Autodesk Inventor part; units mm, degrees
ref_plane "YZ Plane" through (0, 0, 0) normal (1, 0, 0) x (0, 1, 0)
ref_plane "XZ Plane" through (0, 0, 0) normal (0, 1, 0) x (-1, 0, 0)
ref_plane "XY Plane" through (0, 0, 0) normal (0, 0, 1) x (1, 0, 0)
sketch "Sketch1" plane through (0, 0, 0) normal (0, 0, 1) x (1, 0, 0)
  circle A0 centre (0, 0) radius 11.25
  circle A1 centre (0, 0) radius 37.0304
  arc A2 (-32.7929, -17.201) -> (-31.2929, -19.799) centre (0, 0) ccw
  line L0 (-32.7929, -17.201) -> (-31.0547, -16.1974)
  line L1 (-32.7929, -17.201) -> (-31.0547, -16.1974)
  line L2 (-29.5547, -18.7955) -> (-31.2929, -19.799)
  line L3 (-31.2929, -19.799) -> (-29.5547, -18.7955)
  line L4 (-16.1974, -31.0547) -> (-17.201, -32.7929)
  line L5 (-17.201, -32.7929) -> (-16.1974, -31.0547)
  arc A3 (-19.799, -31.2929) -> (-17.201, -32.7929) centre (0, 0) ccw
  line L6 (-19.799, -31.2929) -> (-18.7955, -29.5547)
  line L7 (-19.799, -31.2929) -> (-18.7955, -29.5547)
  arc A4 (17.201, -32.7929) -> (19.799, -31.2929) centre (0, 0) ccw
  line L8 (17.201, -32.7929) -> (16.1974, -31.0547)
  line L9 (17.201, -32.7929) -> (16.1974, -31.0547)
  line L10 (18.7955, -29.5547) -> (19.799, -31.2929)
  line L11 (19.799, -31.2929) -> (18.7955, -29.5547)
  arc A5 (31.2929, -19.799) -> (32.7929, -17.201) centre (0, 0) ccw
  line L12 (31.2929, -19.799) -> (29.5547, -18.7955)
  line L13 (31.0547, -16.1974) -> (32.7929, -17.201)
  line L14 (32.7929, -17.201) -> (31.0547, -16.1974)
  line L15 (32.7929, 17.201) -> (31.0547, 16.1974)
  line L16 (32.7929, 17.201) -> (31.0547, 16.1974)
  arc A6 (32.7929, 17.201) -> (31.2929, 19.799) centre (0, 0) ccw
  line L17 (29.5547, 18.7955) -> (31.2929, 19.799)
  line L18 (31.2929, 19.799) -> (29.5547, 18.7955)
  line L19 (16.1974, 31.0547) -> (17.201, 32.7929)
  line L20 (17.201, 32.7929) -> (16.1974, 31.0547)
  line L21 (19.799, 31.2929) -> (18.7955, 29.5547)
  line L22 (19.799, 31.2929) -> (18.7955, 29.5547)
  line L23 (-17.201, 32.7929) -> (-16.1974, 31.0547)
  line L24 (-17.201, 32.7929) -> (-16.1974, 31.0547)
  line L25 (-18.7955, 29.5547) -> (-19.799, 31.2929)
  line L26 (-19.799, 31.2929) -> (-18.7955, 29.5547)
  arc A7 (-31.2929, 19.799) -> (-32.7929, 17.201) centre (0, 0) ccw
  line L27 (-31.2929, 19.799) -> (-29.5547, 18.7955)
  line L28 (-31.2929, 19.799) -> (-29.5547, 18.7955)
  line L29 (-31.0547, 16.1974) -> (-32.7929, 17.201)
  line L30 (-32.7929, 17.201) -> (-31.0547, 16.1974)
  arc A8 (-21.806, -27.4089) -> (-27.4089, -21.806) centre (-22.4506, -22.4506) ccw
  circle A9 centre (-31.75, 0) radius 5
  arc A10 (-3.9618, 34.8002) -> (-2.3096, 31.8679) centre (-22.4506, 22.4506) ccw
  circle A11 centre (-22.4506, 22.4506) radius 5
  circle A12 centre (22.4506, 22.4506) radius 5
  circle A13 centre (22.4506, 22.4506) radius 5
  arc A14 (-3.9618, -34.8002) -> (-1.7951, -38.6456) centre (22.4506, -22.4506) ccw
  circle A15 centre (22.4506, -22.4506) radius 5
  circle A16 centre (-22.4506, 22.4506) radius 4.75
  circle A17 centre (-22.4506, -22.4506) radius 4.75
  circle A18 centre (22.4506, -22.4506) radius 4.75
  circle A19 centre (22.4506, 22.4506) radius 4.75
  circle A20 centre (0, 0) radius 34.775
  circle A21 centre (0, 0) radius 36.75
  point P0 (0, 0)
  point P1 (0, 49.75)
  point P2 (27.1463, 21.7343)
  point P3 (21.7343, 27.1463)
  point P4 (-21.7343, 27.1463)
  point P5 (-27.1463, 21.7343)
  point P6 (-27.1463, -21.7343)
  point P7 (-21.7343, -27.1463)
  point P8 (21.7343, -27.1463)
  point P9 (27.1463, -21.7343)
  dimension "d6" = 70.05
  dimension "d8" = 74.0608
  dimension "d0" = 10
  dimension "d1" = 0.25
  dimension "d4" = 360
  dimension "d7" = 0.25
  dimension "d9" = 73.5
extrude "Extrusion1" add sketch "Sketch1" along normal blind 21.9 contours A0 A10 | A9 A20 A11 A12 A15 A8 | A9 A20 A10 | A10 A20 A9 | A10 A0 | A20 A16 A11 | A8 A20 A17 | A20 A16 | A16 A20 | A20 A17 | A17 A20 | A15 A20 A18 | A20 A19 A12 | A20 A18 | A18 A20 | A20 A19 | A19 A20 picked at (-31.3962, -1.5997) picked at (-30.2693, 2.6951) picked at (-26.6756, 20.1619) picked at (20.1869, -26.6901) picked at (20.1869, 26.6901)
sketch "Skizze6" plane through (0, 0, 21.9) normal (0, 0, 1) x (1, 0, 0)
  circle A0 centre (0, 0) radius 12.225
  dimension "d33" = 24.45
extrude "Extrusion6" cut sketch "Skizze6" against normal through all
sketch "Skizze7" plane through (0, 0, 21.9) normal (0, 0, 1) x (1, 0, 0)
  line L0 (0, 0) -> (0, 1.75)
  line L1 (-25.23, 24.52) -> (25.23, 24.52)
  line L2 (25.23, 24.52) -> (25.23, -21.02)
  line L3 (25.23, -21.02) -> (-25.23, -21.02)
  line L4 (-25.23, -21.02) -> (-25.23, 24.52)
  line L5 (-25.23, 24.52) -> (25.23, -21.02) construction
  line L6 (25.23, 24.52) -> (-25.23, -21.02) construction
  dimension "d48" = 1.75
  dimension "d49" = 50.46
  dimension "d50" = 45.54
extrude "Extrusion7" cut sketch "Skizze7" against normal blind 7.4
sketch "Skizze8" plane through (0, 0, 0) normal (0, 0, -1) x (-1, 0, 0)
  circle A0 centre (0, 0) radius 12.225
  line L0 (-11.57, 11.47) -> (11.57, 11.47)
  line L1 (11.57, 11.57) -> (11.57, -11.57)
  line L2 (11.57, -11.57) -> (-11.57, -11.57)
  line L3 (-11.57, -11.57) -> (-11.57, 11.57)
  line L4 (-11.57, 11.57) -> (11.57, -11.57) construction
  line L5 (11.57, 11.57) -> (-11.57, -11.57) construction
  circle A1 centre (-11.57, 11.47) radius 1.75
  circle A2 centre (11.57, 11.47) radius 1.75
  circle A3 centre (11.57, -11.57) radius 1.75
  circle A4 centre (-11.57, -11.57) radius 1.75
  dimension "d40" = 23.14
  dimension "d41" = 23.14
  dimension "d42" = 3.5
  dimension "d43" = 3.5
  dimension "d44" = 3.5
  dimension "d45" = 3.5
extrude "Extrusion8" cut sketch "Skizze8" against normal through all contours A2 L0 L1 | L1 L0 A2 | A3 L2 L1 | L1 L2 A3 | A1 L3 L0 | L0 L3 A1 | A4 L3 L2 | L2 L3 A4
sketch "Skizze9" plane through (0, 0, 0) normal (0, 0, -1) x (-1, 0, 0)
  circle A0 centre (-11.57, 11.47) radius 1.75
  circle A1 centre (11.57, 11.47) radius 1.75
  circle A2 centre (11.57, -11.57) radius 1.75
  circle A3 centre (-11.57, -11.57) radius 1.75
  circle A4 centre (-11.57, 11.47) radius 3.1
  circle A5 centre (11.57, 11.47) radius 3.1
  circle A6 centre (11.57, -11.57) radius 3.1
  circle A7 centre (-11.57, -11.57) radius 3.1
  point P0 (0, 0)
  dimension "d51" = 6.2
  dimension "d52" = 6.2
  dimension "d53" = 6.2
  dimension "d54" = 6.2
extrude "Extrusion9" cut sketch "Skizze9" against normal blind 3.5 contours A0 | A1 | A2 | A3 | A4 | A5 | A6 | A7
properties part number "2024_08_26_beam_combiner_blende"
Verification items for the finished model (mm, model axes). A direction names the side the tool comes from. Coordinates: 2 decimals unless noted, no trailing zeros. Write each loop counter-clockwise with the first axis right and the second up, starting at its lowest first coordinate (ties: lowest second). Pieces come first, ordered by that corner, then holes. Notation, with made-up numbers: (80, -31.75) - (97, -31.75) arc R16 ccw to (97, -24.75) - close; hole circle Ø2 at (87, 20.5). An arc over 180 degrees is marked (long way). Write item = value, one per line.
Q1. Cross-section at C-C (x = 0). Enter the section's corners in (y, z) (3 decimals).
Answer:
outline = (-34.775, 0) - (-12.225, 0) - (-12.225, 14.5) - (-21.02, 14.5) - (-21.02, 21.9) - (-34.775, 21.9) - close; (12.225, 0) - (34.775, 0) - (34.775, 21.9) - (24.52, 21.9) - (24.52, 14.5) - (12.225, 14.5) - close
Q2. Cross-section at D-D (z = 16.75). Enter the section's corners in (x, y) (3 decimals), plus the area to 3 significant figures.
Answer:
outline = (-27.146, -21.734) arc R4.75 ccw to (-21.734, -27.146) arc R34.775 ccw to (21.734, -27.146) arc R4.75 ccw to (27.146, -21.734) arc R34.775 ccw to (27.146, 21.734) arc R4.75 ccw to (21.734, 27.146) arc R34.775 ccw to (-21.734, 27.146) arc R4.75 ccw to (-27.146, 21.734) arc R34.775 ccw to start; hole (-25.23, -21.02) - (25.23, -21.02) - (25.23, 24.52) - (-25.23, 24.52) - close
area = 1,540 mm²
Q3. Access from +Z, -Z, +X, -X, +Y, -Y to the whole of each face (thin tool, end or side, straight path). Record for faces 1 (the face through (0, -23, 21.9)), 2 (the face through (10.14, 8.72, 1.73)), 3 (the face through (0, -21.02, 18)).
Answer:
face_1 = +Z, +X, -X, +Y, -Y
face_2 = -Z
face_3 = +Z
Q4. Cross-section at A-A (y = 0). Enter the section's corners in (x, z) (3 decimals), plus the area to 3 significant figures.
Answer:
outline = (-34.775, 0) - (-12.225, 0) - (-12.225, 14.5) - (-25.23, 14.5) - (-25.23, 21.9) - (-34.775, 21.9) - close; (12.225, 0) - (34.775, 0) - (34.775, 21.9) - (25.23, 21.9) - (25.23, 14.5) - (12.225, 14.5) - close
area = 795 mm²
Q5. Go/stop test with flat-tipped pins: pin 1 Ø5 at (x, y) = (6, 12.5) entering from +Z; pin 2 Ø6 at (x, z) = (-13, 11) entering from -Y; pin 3 Ø3 at (y, z) = (-11.5, 5.5) entering from -X; pin 4 Ø7 at (x, y) = (11.57, 11.47) entering from -Z. Record where each tip stops, or that it passes through.
Answer:
pin_1 = 14.5
pin_2 = -33.31
pin_3 = -33.31
pin_4 = 0
Q6. Material ranges on L1, parallel to Y at x = 0.5, z = 3.25; L2, parallel to Y at x = -13, z = 4; L3, parallel to Y at x = 7, z = 5.5, recorded low to high. Write a range as from..to.
Answer:
L1 = -34.77..-12.21, 12.21..34.77
L2 = -32.25..-12.58, -10.56..10.46, 12.48..32.25
L3 = -34.06..-10.02, 10.02..34.06
Q7. Cross-section at B-B (z = 10.25). Enter the section's corners in (x, y) (3 decimals).
Answer:
outline = (-27.146, -21.734) arc R4.75 ccw to (-21.734, -27.146) arc R34.775 ccw to (21.734, -27.146) arc R4.75 ccw to (27.146, -21.734) arc R34.775 ccw to (27.146, 21.734) arc R4.75 ccw to (21.734, 27.146) arc R34.775 ccw to (-21.734, 27.146) arc R4.75 ccw to (-27.146, 21.734) arc R34.775 ccw to start; hole circle Ø3.5 at (-11.57, -11.57); hole circle Ø3.5 at (-11.57, 11.47); hole circle Ø24.45 at (0, 0); hole circle Ø3.5 at (11.57, -11.57); hole circle Ø3.5 at (11.57, 11.47)
Q8. Mould release check, pull along X, two halves, no side actions. Record for faces 4 (the face through (-34.773, -0.329, 10.797)), 5 (the face through (0.329, -34.773, 10.797)), 6 (the face through (-10.898, 8.444, 1.726)): released by +X, released by -X, zero draft, split by the parting line, or undercut.
Answer:
face_4 = released by -X
face_5 = split by the parting line
face_6 = undercut
